Verification items for the finished model (mm, model axes). Coordinates: 2 decimals unless noted, no trailing zeros. Loops run counter-clockwise (first coordinate to the right, second up) from the corner with the lowest first, then second, coordinate; pieces in that order, holes last. Notation, with made-up numbers: M 27,-25.75 L 50,-25.75 A18 cw 50,-1.75 Z; hole C 86.5,65 d3. An arc over 180 degrees is marked long. Write item = value, one per line. Start each with the question number.
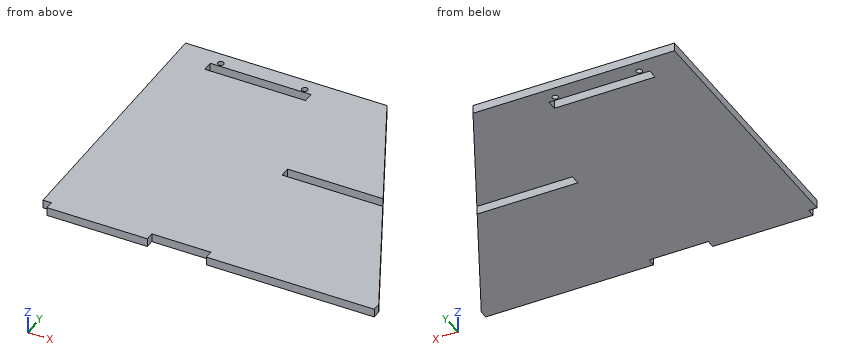
```python
from build123d import *

# Parameters (mm, degrees)
SKETCH1_W           = 100
SKETCH1_H           = 5
SKETCH1_W_2         = 59.8
BOSS_EXTRUDE1_DEPTH = 5
SKETCH2_W           = 60
SKETCH2_H           = 6.1
CUT_EXTRUDE1_DEPTH  = 5
SKETCH3_R           = 1.75
CUT_EXTRUDE2_DEPTH  = 5
SKETCH4_W           = 60
SKETCH4_H           = 6.1
CUT_EXTRUDE3_DEPTH  = 5


with BuildPart() as part:
    # Sketch1 → Boss-Extrude1 (new body)
    with BuildSketch(Plane.XY):
        Polygon((120, 160), (200, 0), (0, 0), (0, 160), align=None)
        with Locations((150, -2.5)):
            Rectangle(SKETCH1_W, SKETCH1_H)
        with Locations((34.9, -2.5)):
            Rectangle(SKETCH1_W_2, SKETCH1_H)
    extrude(amount=BOSS_EXTRUDE1_DEPTH)

    # Sketch2 → Cut-Extrude1 (cut)
    with BuildSketch(Plane.XY.offset(5)):
        with Locations((50, 146.95)):
            Rectangle(SKETCH2_W, SKETCH2_H)
    extrude(amount=-CUT_EXTRUDE1_DEPTH, mode=Mode.SUBTRACT)

    # Sketch3 → Cut-Extrude2 (cut)
    with BuildSketch(Plane.XY.offset(5)):
        with Locations((25, 152.5)):
            Circle(SKETCH3_R)
        with Locations(Location((75, 152.5, 0), (0, 0, 180))):
            Circle(SKETCH3_R)
    extrude(amount=-CUT_EXTRUDE2_DEPTH, mode=Mode.SUBTRACT)

    # Sketch4 → Cut-Extrude3 (cut)
    with BuildSketch(Plane.XY.offset(5)):
        with Locations((130.55, 81.95)):
            Rectangle(SKETCH4_W, SKETCH4_H)
    extrude(amount=-CUT_EXTRUDE3_DEPTH, mode=Mode.SUBTRACT)


solid = part.part
```
Q1. Sectioned sample at C-C on x = 178. Record the cut outline in (y, z).
Q2. Sectioned sample at B-B on y = 68. Record the cut outline in (x, z), plus the area to 3 significant figures.
Q3. Gauge pin test, flat ends, axial feed: pin 1 (5.5 mm diameter, centred on x = 25, y = 152.5, fed in from -Z); pin 2 (1.5 mm diameter, centred on x = 2.5, z = 3.5, fed in from -Y); pin 3 (2.5 mm diameter, centred on x = 139.5, z = 1.5, fed in from +Y); pin 4 (2.5 mm diameter, centred on y = -2, z = 2.5, fed in from -X). Record the tip position at first contact, or that the pin passes through.
Q4. Scan lines: L1, parallel to Y at x = 75, z = 3; L2, parallel to Y at x = 25, z = 2; L3, parallel to Y at x = 66, z = 3.3. Record each from-to range of solid material in increasing order. Write a range as [from, to].
Q5. Sectioned sample at A-A on z = 3.15. Record the cut outline in (x, y), plus the area to 3 significant figures.
Solutions:
q1.outline = M -5,0 L 44,0 L 44,5 L -5,5 Z
q2.outline = M 0,0 L 166,0 L 166,5 L 0,5 Z
q2.area = 830 mm²
q3.pin_1 = 0
q3.pin_2 = 0
q3.pin_3 = 123.5
q3.pin_4 = 5
q4.L1 = [0, 143.9], [150, 150.75], [154.25, 160]
q4.L2 = [-5, 143.9], [150, 150.75], [154.25, 160]
q4.L3 = [0, 143.9], [150, 160]
q5.outline = M 0,0 L 5,0 L 5,-5 L 64.8,-5 L 64.8,0 L 100,0 L 100,-5 L 200,-5 L 200,0 L 160.55,78.9 L 100.55,78.9 L 100.55,85 L 157.5,85 L 120,160 L 0,160 Z; hole M 20,143.9 L 80,143.9 L 80,150 L 20,150 Z; hole C 25,152.5 d3.5; hole C 75,152.5 d3.5
q5.area = 25,700 mm²
